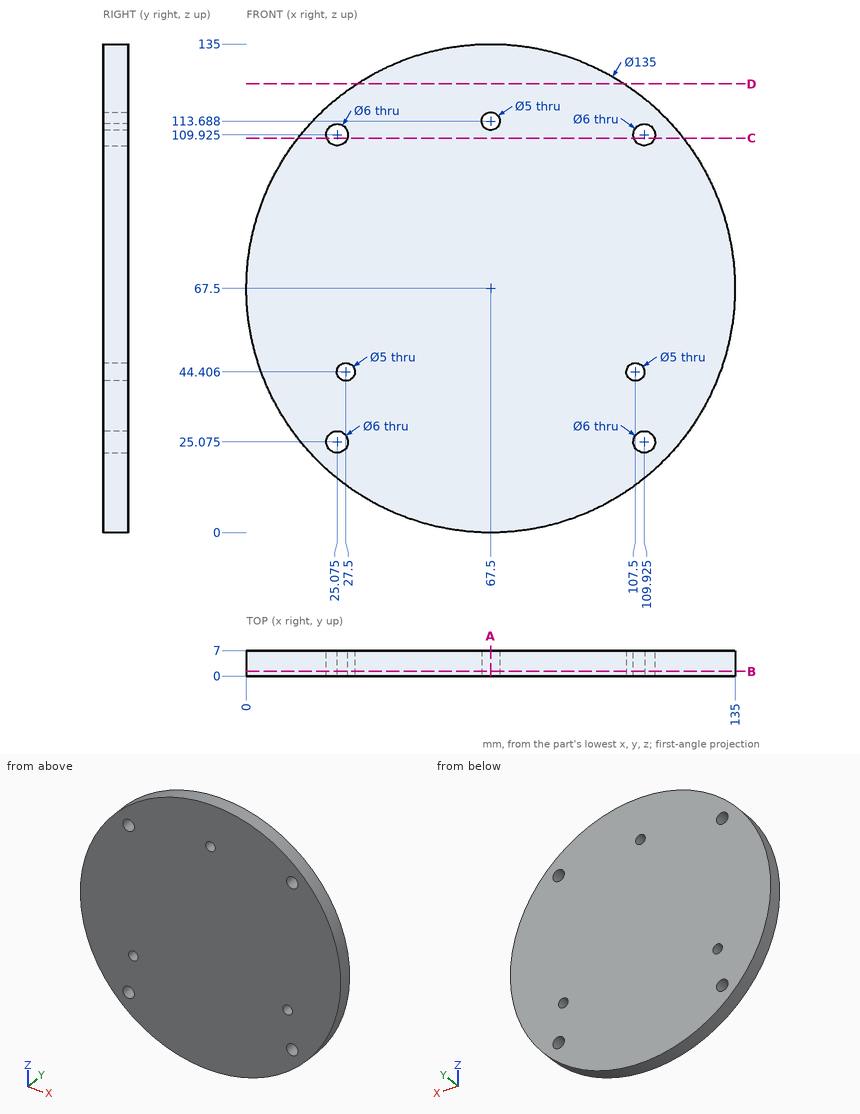
Geometry check sheet. Reference: drawing and pictorial views, mm from the part's lowest x, y, z. Give positions to 0.01 mm unless a question says otherwise; leave off trailing zeros. Loops run counter-clockwise (first coordinate to the right, second up) from the corner with the lowest first, then second, coordinate; pieces in that order, holes last. Notation, with made-up numbers: (54, 60.25) - (93, 60.25) arc R35 ccw to (93, 98.25) - close; hole circle Ø5 at (-10.75, 44). An arc over 180 degrees is marked (long way). One line per question, with ' | ' between items. Start each with the question number.
1. Cross-section at C-C, the plane z = 109. Enter the section's corners in (x, y).
2. Cross-section at B-B, the plane y = 1.25. Enter the section's corners in (x, z) (3 decimals), plus the area to 3 significant figures.
3. Material ranges on line 1 along X through (y, z) = (2.5, 110.5); line 2 along Z through (x, y) = (108.5, 5) (3 decimals); line 3 along X through (y, z) = (1.25, 109), recorded low to high. Write a range as [from, to].
4. Gauge pin test, flat ends, axial feed: pin 1 Ø1 at (y, z) = (1, 27) entering from -X; pin 2 Ø3.5 at (x, z) = (109.925, 25.075) entering from -Y (1 decimal). Record the tip position at first contact, or that the pin passes through.
5. Cross-section at D-D, the plane z = 124. Enter the section's corners in (x, y).
6. Cross-section at A-A, the plane x = 67.5. Enter the section's corners in (y, z), plus the area to 3 significant figures.
Check result:
1) outline: (14.26, 0) - (22.22, 0) - (22.22, 7) - (14.26, 7) - close; (27.93, 0) - (107.07, 0) - (107.07, 7) - (27.93, 7) - close; (112.78, 0) - (120.74, 0) - (120.74, 7) - (112.78, 7) - close
2) outline: circle Ø135 at (67.5, 67.5); hole circle Ø6 at (25.075, 25.075); hole circle Ø6 at (25.075, 109.925); hole circle Ø5 at (27.5, 44.406); hole circle Ø5 at (67.5, 113.688); hole circle Ø5 at (107.5, 44.406); hole circle Ø6 at (109.925, 25.075); hole circle Ø6 at (109.925, 109.925) | area: 14,100 mm2
3) line 1: x = [15.47, 22.13], [28.02, 106.98], [112.87, 119.53] | line 2: z = [13.879, 22.435], [27.715, 42.115], [46.697, 107.285], [112.565, 121.121] | line 3: x = [14.26, 22.22], [27.93, 107.07], [112.78, 120.74]
4) pin 1: stops at x = 13.13 | pin 2: passes through
5) outline: (30.57, 0) - (104.43, 0) - (104.43, 7) - (30.57, 7) - close
6) outline: (0, 0) - (7, 0) - (7, 111.19) - (0, 111.19) - close; (0, 116.19) - (7, 116.19) - (7, 135) - (0, 135) - close | area: 910 mm2
